CAD build for the part. Positions are in the model's coordinates, mm. Coordinates: 2 decimals unless noted, no trailing zeros. Loops run counter-clockwise (first coordinate to the right, second up) from the corner with the lowest first, then second, coordinate; pieces in that order, holes last.
1) Wall check: line 1 along Z through (x, y) = (-65.5, -12); line 2 along X through (y, z) = (6.5, -513); line 3 along Y through (x, z) = (-11, -739). Give the ranges that are in metal, low to high.
2) Saw through at B-B, the plane z = -2269. Write the cut outline in (x, y).
3) Saw through at A-A, the plane x = -59. Write the cut outline in (y, z).
4) Pin check, flat tips, straight feed: pin 1 Ø12 at (y, z) = (23.5, -2215.5) entering from +X; pin 2 Ø4 at (x, y) = (-37.5, -7) entering from -Z. Stop position of each tip, or through.
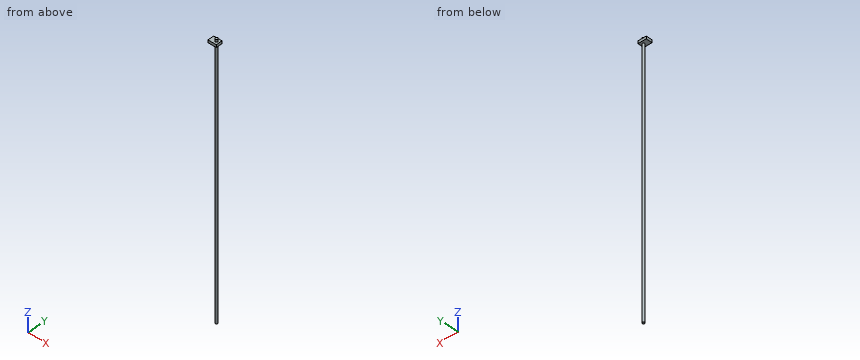
```python
from build123d import *

# Parameters (mm, degrees)
F0_W          = 80.712397
F0_H          = 59.831567
F1_DEPTH      = 25.4
F2_R          = 11.951045
F3_DEPTH      = 25.4
F3_DEPTH_BACK = 2540


with BuildPart() as f1:
    # F0 (on Top) → F1 (new body)
    with BuildSketch(Plane.XY):
        with Locations((-35.909553, 8.104238)):
            Rectangle(F0_W, F0_H)
    extrude(amount=F1_DEPTH)

    # F2 (on face) → F3 (join, two sides)
    with BuildSketch(Plane.XY.offset(25.4)) as f3_sk:
        with Locations((-21.637337, 8.478672)):
            Circle(F2_R)
    extrude(amount=F3_DEPTH)
    extrude(f3_sk.sketch, amount=-F3_DEPTH_BACK)


solid = f1.part
```
Data:
1. line 1: z = 0 to 25.4
1. line 2: x = -33.42 to -9.85
1. line 3: y = 3.03 to 13.93
2. outline: circle Ø23.9 at (-21.64, 8.48)
3. outline: (-21.81, 0) - (38.02, 0) - (38.02, 25.4) - (-21.81, 25.4) - close
4. pin 1: stops at x = -13.8
4. pin 2: stops at z = 0
